from build123d import *

# Parameters (mm, degrees)
SKETCH4_R               = 1.875
BOSS_EXTRUDE2_DEPTH     = 1.5
SKETCH5_OUTSIDE_W       = 61.376
SKETCH5_OUTSIDE_H       = 60.602
SKETCH5_OUTSIDE_R       = 2.5
CUT_EXTRUDE1_DEPTH      = 15
CUT_EXTRUDE1_DRAFT      = -60
MIRROR1_COPY_1_SKETCH_W = 61.376
MIRROR1_COPY_1_SKETCH_H = 60.602
MIRROR1_COPY_1_SKETCH_R = 2.5
MIRROR1_COPY_1_DEPTH    = 15
MIRROR1_COPY_1_DRAFT    = -60
SKETCH4_3_R             = 1.875
BOSS_EXTRUDE3_DEPTH     = 10
FILLET1_R               = 1
FILLET2_R               = 0.5


with BuildPart() as part:
    # Sketch4 → Boss-Extrude2 (new, symmetric)
    with BuildSketch(Plane.XY):
        Polygon((2.886751346, 0), (1.443375673, 2.5), (-1.443375673, 2.5), (-2.886751346, 0), (-1.443375673, -2.5), (1.443375673, -2.5), align=None)
        Circle(SKETCH4_R, mode=Mode.SUBTRACT)
        Circle(SKETCH4_R)
    extrude(amount=BOSS_EXTRUDE2_DEPTH, both=True)


with BuildPart() as cut_extrude1_tool:
    # Sketch5 outside → Cut-Extrude1 (with draft: the straight prism first)
    with BuildSketch(Plane.XY.offset(1.5)):
        Rectangle(SKETCH5_OUTSIDE_W, SKETCH5_OUTSIDE_H)
        Circle(SKETCH5_OUTSIDE_R, mode=Mode.SUBTRACT)
    extrude(amount=-CUT_EXTRUDE1_DEPTH)
    # Cut-Extrude1: the draft: its side faces are tilted about the plane it starts from
    cut_extrude1_sides = [cut_extrude1_tool.faces().sort_by_distance(p)[0] for p in [
        (0, -30.301, -6),
        (30.688, 0, -6),
        (0, 30.301, -6),
        (-30.688, 0, -6),
        (-2.5, 0, -6),
    ]]
    draft(cut_extrude1_sides, Plane.XY.offset(1.5), CUT_EXTRUDE1_DRAFT)


with BuildPart() as part_1:
    add(part.part)

    # Cut-Extrude1: cut by cut_extrude1_tool
    add(cut_extrude1_tool.part, mode=Mode.SUBTRACT)


with BuildPart() as mirror1_copy_1_tool:
    # Mirror1 copy 1 sketch → Mirror1 copy 1 (with draft: the straight prism first)
    with BuildSketch(Plane(origin=(0, 0, -1.5), x_dir=(1, 0, 0), z_dir=(0, 0, -1))):
        Rectangle(MIRROR1_COPY_1_SKETCH_W, MIRROR1_COPY_1_SKETCH_H)
        Circle(MIRROR1_COPY_1_SKETCH_R, mode=Mode.SUBTRACT)
    extrude(amount=-MIRROR1_COPY_1_DEPTH)
    # Mirror1 copy 1: the draft: its side faces are tilted about the plane it starts from
    mirror1_copy_1_sides = [mirror1_copy_1_tool.faces().sort_by_distance(p)[0] for p in [
        (0, -30.301, 6),
        (30.688, 0, 6),
        (0, 30.301, 6),
        (-30.688, 0, 6),
        (-2.5, 0, 6),
    ]]
    draft(mirror1_copy_1_sides, Plane(origin=(0, 0, -1.5), x_dir=(1, 0, 0), z_dir=(0, 0, -1)), MIRROR1_COPY_1_DRAFT)


with BuildPart() as part_2:
    add(part_1.part)

    # Mirror1 copy 1: cut by mirror1_copy_1_tool
    add(mirror1_copy_1_tool.part, mode=Mode.SUBTRACT)

    # Sketch4_3 → Boss-Extrude3 (add)
    with BuildSketch(Plane.XY):
        Circle(SKETCH4_3_R)
    extrude(amount=BOSS_EXTRUDE3_DEPTH)

    # Fillet1
    fillet1_edges = [part_2.edges().sort_by_distance(p)[0] for p in [
        (2.886751346, 0, 0),
        (1.443375673, -2.5, 0),
        (-1.443375673, -2.5, 0),
        (-2.886751346, 0, 0),
        (-1.443375673, 2.5, 0),
        (1.443375673, 2.5, 0),
    ]]
    fillet(fillet1_edges, radius=FILLET1_R)

    # Fillet2
    fillet2_edges = [part_2.edges().sort_by_distance(p)[0] for p in [
        (-1.875, 0, 10),
    ]]
    fillet(fillet2_edges, radius=FILLET2_R)


solid = part_2.part
Work out the finished part from the listing and answer in its coordinate system (mm). A direction names the side the tool comes from. Round coordinates to 2 decimals unless told otherwise and drop trailing zeros. Write each loop counter-clockwise with the first axis right and the second up, starting at its lowest first coordinate (ties: lowest second). Pieces come first, ordered by that corner, then holes. Notation, with made-up numbers: (65, 34) -> (98, 34) arc R8 cw to (98, 43) -> close; hole circle Ø5 at (60, 23.5). An arc over 180 degrees is marked (long way). Answer as CSV lines item,"result". Start each with the question number.
(1) Find the intervals of material crossed by probe 1 along Z at (x, y) = (-0.2, -2.15); probe 2 along X at (y, z) = (-1.25, 1); probe 3 along Y at (x, z) = (0.1, 9.5), in increasing order.
(2) The part is cut by section B-B, the plane z = 8. Give the vertices of the cut face in (x, y) (3 decimals), then the cut area to 3 significant figures.
(3) Each of these flat-tipped pins is pushed along its axis until it touches: pin 1 (2 mm diameter, centred on x = -2, z = 0.5, fed in from -Y); pin 2 (1 mm diameter, centred on y = -0.5, z = 4, fed in from -X) (3 decimals); pin 3 (3 mm diameter, centred on x = -1.5, y = 1, fed in from +Z). Where does it stop, or does it pass through?
(4) The part is cut by section A-A, the plane y = 0. Give the vertices of the cut face in (x, z) (3 decimals).
(5) A tool of negligible diameter and unlimited length cuts with its end or side. For faces 1 (the flat face through (2.17, 1.24, 0.02)), 2 (the cylindrical face through (-1.873, 0.082, 5.444)), from which of +Z, -Z, +X, -X, +Y, -Y can it reach the whole face along a straight path? Write none if from no direction.
Output values:
1,probe 1,"z = -1.5 to 1.5"
1,probe 2,"x = -2.17 to 2.17"
1,probe 3,"y = -1.87 to 1.87"
2,outline,"circle Ø3.75 at (0, 0)"
2,area,"11.0 mm²"
3,pin 1,"stops at y = -2.49"
3,pin 2,"stops at x = -1.875"
3,pin 3,"stops at z = 10"
4,outline,"(-2.732, -1.366) -> (-2.5, -1.5) -> (2.5, -1.5) -> (2.732, -1.366) -> (2.732, 1.366) -> (2.5, 1.5) -> (1.875, 1.5) -> (1.875, 9.5) arc R0.5 ccw to (1.375, 10) -> (-1.375, 10) arc R0.5 ccw to (-1.875, 9.5) -> (-1.875, 1.5) -> (-2.5, 1.5) -> (-2.732, 1.366) -> close"
5,face 1,"+Z, -Z, +X, +Y"
5,face 2,"+Z"
